Geometry: final body of the model. Coordinates: model frame, mm. Face numbers are marked on the shaded views. A direction names the side the tool comes from. Give positions to 0.01 mm unless a question says otherwise; leave off trailing zeros. Write each loop counter-clockwise with the first axis right and the second up, starting at its lowest first coordinate (ties: lowest second). Pieces come first, ordered by that corner, then holes.
Q1. Section C-C (y = 5). Return the cut outline in (x, z) (3 decimals), plus the area to 3 significant figures.
Q2. Line query: line 1 (X direction, y = 4.75, z = 0.75); line 2 (Y direction, x = -11, z = -0.25) (3 decimals); line 3 (X direction, y = 6.25, z = 1.75). Output: solid intervals per line, ascending.
Q3. Section D-D (z = -4). Return the cut outline in (x, y) (3 decimals), plus the area to 3 significant figures.
Q4. Reachability of the marked faces 1 and 2 from +Z, -Z, +X, -X, +Y, -Y: full face, straight path, thin tool, end or side. Return the list, or none.
Q5. Pin query (flat end, axial travel): pin 1 Ø1 at (x, z) = (26.5, 5.5) entering from +Y (3 decimals); pin 2 Ø3 at (y, z) = (5.5, -4) entering from +X; pin 3 Ø1.5 at (y, z) = (5.5, 2) entering from -X. Return the tip coordinate at first contact, or that it passes through.
Q6. Section B-B (z = 0.5). State how many separate pieces and enclosed holes the cut face has, plus the area to 3 significant figures.
Q7. Section A-A (y = 1.5). Return the cut outline in (x, z) (3 decimals), plus the area to 3 significant figures.
from build123d import *

# Parameters (mm, degrees)
BOSS_EXTRUDE1_DEPTH = 2.975
SKETCH2_R           = 2.175
CUT_EXTRUDE1_DEPTH  = 12.7
SKETCH3_R           = 2.175
BOSS_EXTRUDE2_DEPTH = 3.775


with BuildPart() as part:
    # Sketch1 → Boss-Extrude1 (new body)
    with BuildSketch(Plane(origin=(0, 0, 0), x_dir=(1, 0, 0), z_dir=(0, 1, 0))):
        with BuildLine():
            Line((-23.171929825, 5.625877193), (43.628070175, 5.625877193))
            ThreePointArc((43.628070175, 5.625877193), (49.978070175, -0.724122807), (43.628070175, -7.074122807))
            Line((43.628070175, -7.074122807), (-23.171929825, -7.074122807))
            ThreePointArc((-23.171929825, -7.074122807), (-29.521929825, -0.724122807), (-23.171929825, 5.625877193))
        make_face()
    extrude(amount=BOSS_EXTRUDE1_DEPTH)

    # Sketch2 → Cut-Extrude1 (cut)
    with BuildSketch(Plane(origin=(0, 2.975, 0), x_dir=(1, 0, 0), z_dir=(0, 1, 0))):
        with Locations(Location((-23.171929825, -0.724122807, 0), (0, 0, 270))):
            Circle(SKETCH2_R)
        with Locations(Location((43.628070175, -0.724122807, 0), (0, 0, 270))):
            Circle(SKETCH2_R)
    extrude(amount=-CUT_EXTRUDE1_DEPTH, mode=Mode.SUBTRACT)

    # Sketch3 → Boss-Extrude2 (add)
    with BuildSketch(Plane(origin=(0, 2.975, 0), x_dir=(1, 0, 0), z_dir=(0, 1, 0))):
        with BuildLine():
            ThreePointArc((43.628070175, 5.625877193), (49.978070175, -0.724122807), (43.628070175, -7.074122807))
            ThreePointArc((43.628070175, -7.074122807), (37.278070175, -0.724122807), (43.628070175, 5.625877193))
        make_face()
        with Locations(Location((43.628070175, -0.724122807, 0), (0, 0, 270))):
            Circle(SKETCH3_R, mode=Mode.SUBTRACT)
    extrude(amount=BOSS_EXTRUDE2_DEPTH)


solid = part.part
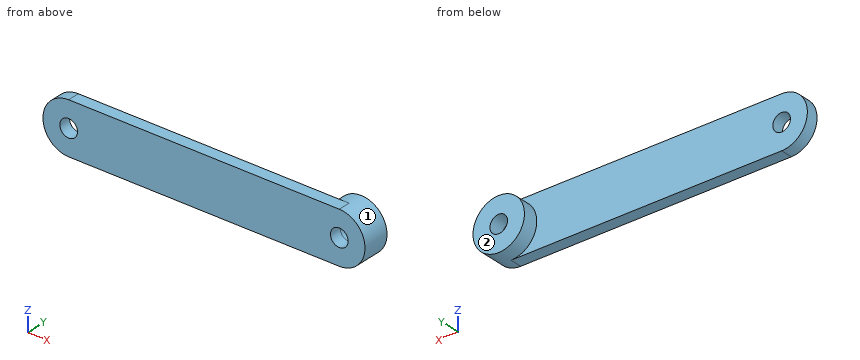
Computed:
1. outline: circle Ø12.7 at (43.628, 0.724); hole circle Ø4.35 at (43.628, 0.724)
1. area: 112 mm2
2. line 1: x = 37.28 to 41.45, 45.8 to 49.98
2. line 2: y = 0 to 2.975
2. line 3: x = 37.36 to 41.71, 45.55 to 49.89
3. outline: (-27.415, 0) - (47.871, 0) - (47.871, 6.75) - (39.385, 6.75) - (39.385, 2.975) - (-27.415, 2.975) - close
3. area: 256 mm2
4. face 1: +Y
4. face 2: +Z, -Z, +X, -X, +Y
5. pin 1: stops at y = 2.975
5. pin 2: stops at x = 49.1
5. pin 3: stops at x = 37.3
6. separate pieces: 3
6. enclosed holes: 0
6. area: 242 mm2
7. outline: (-23.172, -5.626) - (43.628, -5.626) arc R6.35 ccw to (43.628, 7.074) - (-23.172, 7.074) arc R6.35 ccw to start; hole circle Ø4.35 at (-23.172, 0.724); hole circle Ø4.35 at (43.628, 0.724)
7. area: 945 mm2
